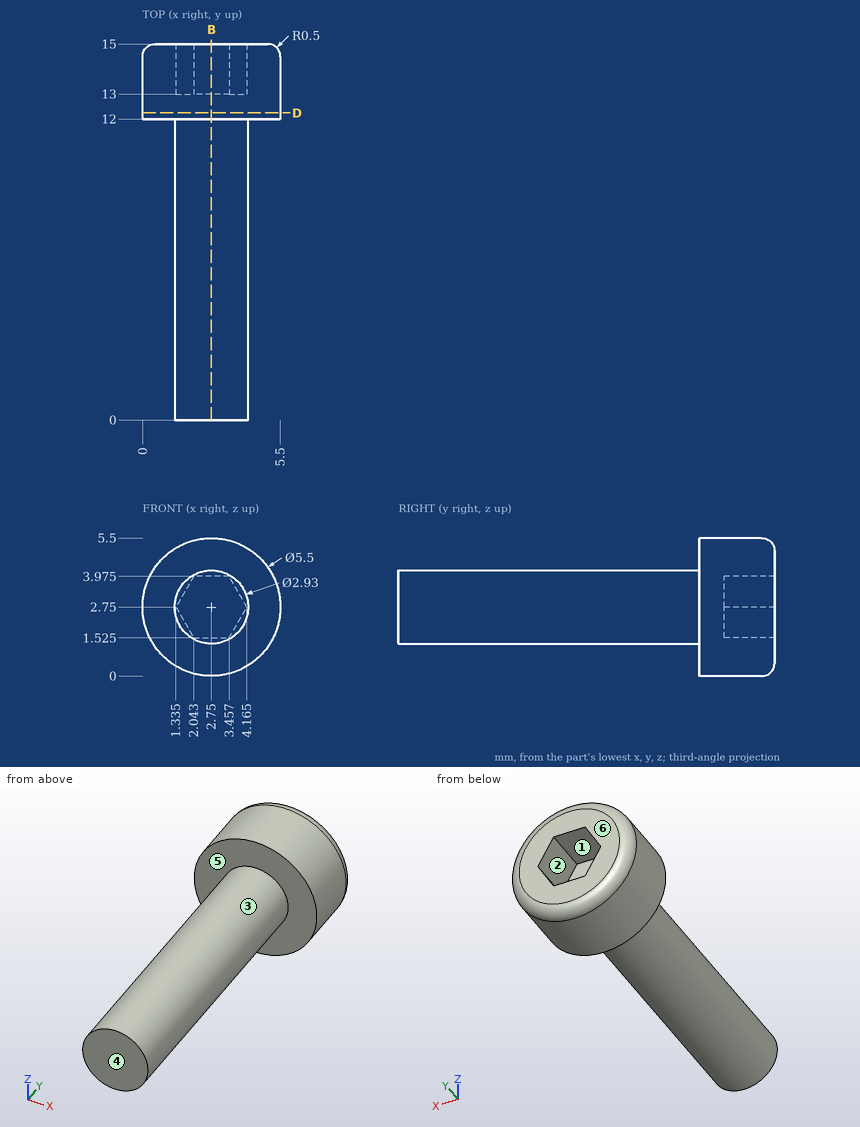
Input: dimensioned drawing with shaded views. Units: mm. Origin: part minimum x, y, z. A direction names the side the tool comes from. Round coordinates to 2 decimals unless told otherwise and drop trailing zeros. Loops run counter-clockwise (first coordinate to the right, second up) from the corner with the lowest first, then second, coordinate; pieces in that order, holes last.
1) Pull-direction query (X, two-part tool) for the marked faces 1, 2, 3 and 4; classes: released by +X, released by -X, zero draft, split by the parting line, or undercut.
Ans:
face 1: undercut
face 2: undercut
face 3: split by the parting line
face 4: zero draft
2) Section query B-B on x = 2.75. Return the cut outline in (y, z) (1 decimal).
Ans:
outline: (0, 1.3) - (12, 1.3) - (12, 0) - (14.5, 0) arc R0.5 ccw to (15, 0.5) - (15, 1.5) - (13, 1.5) - (13, 4) - (15, 4) - (15, 5) arc R0.5 ccw to (14.5, 5.5) - (12, 5.5) - (12, 4.2) - (0, 4.2) - close
3) Section query D-D on y = 12.25. Return the cut outline in (x, z).
Ans:
outline: circle Ø5.5 at (2.75, 2.75)
4) Material intervals for line 1 (Y direction, x = 1.3, z = 1.45); line 2 (Z direction, x = 2.85, y = 10); line 3 (Z direction, x = 2.7, y = 13.5) (1 decimal), sorted ascending.
Ans:
line 1: y = 12 to 15
line 2: z = 1.29 to 4.21
line 3: z = 0 to 1.5, 4 to 5.5
5) Pin query (flat end, axial travel): pin 1 (1.1 mm diameter, centred on x = 2.5, y = 14, fed in from -Z); pin 2 (2 mm diameter, centred on x = 1, y = 2, fed in from -Z); pin 3 (0.7 mm diameter, centred on x = 3, z = 3, fed in from +Y); pin 4 (1 mm diameter, centred on x = 4.5, y = 7.5, fed in from +Z) (1 decimal). Return the tip coordinate at first contact, or that it passes through.
Ans:
pin 1: stops at z = 0
pin 2: stops at z = 1.49
pin 3: stops at y = 13
pin 4: stops at z = 3.5
6) Set-up query: the marked faces 5 and 6. Return all of +Z, -Z, +X, -X, +Y, -Y with unobstructed straight access to the full face (end or side cutting, diameter ignored); none if empty.
Ans:
face 5: -Y
face 6: +Z, -Z, +X, -X, +Y
